Design review of the part built by this model. Coordinates are the model's own, in mm. Face numbers are marked on the shaded views. A direction names the side the tool comes from. Round coordinates to 2 decimals unless told otherwise and drop trailing zeros. Write each loop counter-clockwise with the first axis right and the second up, starting at its lowest first coordinate (ties: lowest second). Pieces come first, ordered by that corner, then holes.
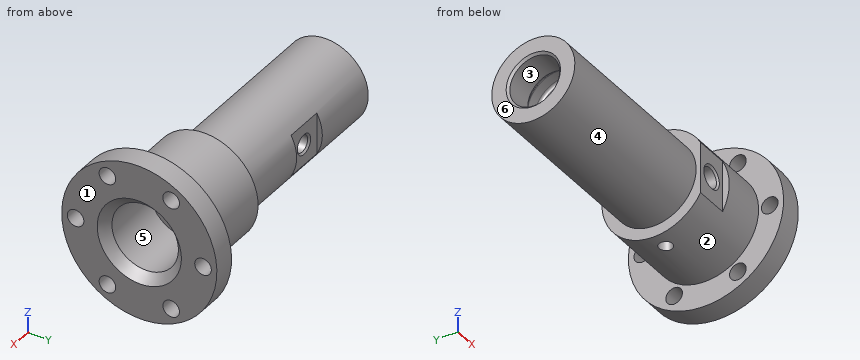
from build123d import *

# Parameters (mm, degrees)
FILLET2_R               = 2.5
SKETCH3_R               = 7.5
CUT_EXTRUDE1_DEPTH      = 274.541587332
CUT_EXTRUDE2_DEPTH      = 181.994025949
CUT_EXTRUDE2_DEPTH_BACK = 181.994025949
SKETCH4_W               = 35
SKETCH4_H               = 5
CUT_EXTRUDE3_DEPTH      = 181.994025949
CUT_EXTRUDE3_DEPTH_BACK = 181.994025949
SKETCH5_W               = 30
SKETCH5_H               = 6
SKETCH6_R               = 7.5
CUT_EXTRUDE4_DEPTH      = 28
SKETCH7_R               = 9
CUT_EXTRUDE5_DEPTH      = 33
CHAMFER6_SIZE           = 1.6
SKETCH8_R               = 6
CUT_EXTRUDE6_DEPTH      = 60


with BuildPart() as part:
    # Sketch1 → Revolve1 (revolve)
    with BuildSketch(Plane.XY, mode=Mode.PRIVATE) as revolve1_sk:
        Polygon((103.47826087, -30), (103.47826087, -70), (83.47826087, -70), (83.47826087, -47.5), (13.47826087, -47.5), (13.47826087, -37.5), (-151.52173913, -37.5), (-151.52173913, -22.5), (-125.02173913, -22.5), (-119.02173913, -27.5), (-106.52173913, -27.5), (-106.52173913, -17.5), (-16.52173913, -17.5), (-16.52173913, -27.5), (-1.52173913, -27.5), (-1.52173913, -22.5), (43.47826087, -22.5), (43.47826087, -30), align=None)
    revolve(revolve1_sk.sketch.rotate(Axis((-977.747346799, 0, 0), (1, 0, 0)), 270), axis=Axis((-977.747346799, 0, 0), (1, 0, 0)))

    # Fillet2
    fillet2_edges = [part.edges().sort_by_distance(p)[0] for p in [
        (-106.52173913, 0, -27.5),
        (-119.02173913, 0, -27.5),
    ]]
    fillet(fillet2_edges, radius=FILLET2_R)

    # Chamfer3: read off the stored shape, not the designer's step
    # Chamfer3 outline → Chamfer3 (revolve, cut)
    with BuildSketch(Plane.YX):
        Polygon((24.5, -151.52173913), (22.5, -149.52173913), (22.5, -151.52173913), align=None)
    revolve(axis=Axis((0, 0, 0), (1, 0, 0)), mode=Mode.SUBTRACT)

    # Chamfer4: read off the stored shape, not the designer's step
    # Chamfer4 outline → Chamfer4 (revolve, cut)
    with BuildSketch(Plane.YX):
        Polygon((30, 103.47826087), (30, 95.47826087), (38, 103.47826087), align=None)
    revolve(axis=Axis((0, 0, 0), (1, 0, 0)), mode=Mode.SUBTRACT)

    # Sketch3 → Cut-Extrude1 (cut, through all)
    with BuildSketch(Plane(origin=(103.47826087, 0, 0), x_dir=(0, 0, -1), z_dir=(1, 0, 0))):
        with Locations((0, 57.5)):
            Circle(SKETCH3_R)
        with Locations((49.796460718, 28.75)):
            Circle(SKETCH3_R)
        with Locations((49.796460718, -28.75)):
            Circle(SKETCH3_R)
        with Locations((0, -57.5)):
            Circle(SKETCH3_R)
        with Locations((-49.796460718, -28.75)):
            Circle(SKETCH3_R)
        with Locations((-49.796460718, 28.75)):
            Circle(SKETCH3_R)
    extrude(amount=-CUT_EXTRUDE1_DEPTH, mode=Mode.SUBTRACT)

    # Sketch4 → Cut-Extrude2 (cut, two sides: drawn at the far end of the back side and taken through both)
    with BuildSketch(Plane.XY.offset(-CUT_EXTRUDE2_DEPTH_BACK)):
        with Locations((-71.52173913, 35)):
            Rectangle(SKETCH4_W, SKETCH4_H)
    extrude(amount=CUT_EXTRUDE2_DEPTH + CUT_EXTRUDE2_DEPTH_BACK, mode=Mode.SUBTRACT)

    # Sketch5 → Cut-Extrude3 (cut, two sides: drawn at the far end of the back side and taken through both)
    with BuildSketch(Plane.XY.offset(-CUT_EXTRUDE3_DEPTH_BACK)):
        with Locations((28.47826087, -44.5)):
            Rectangle(SKETCH5_W, SKETCH5_H)
    extrude(amount=CUT_EXTRUDE3_DEPTH + CUT_EXTRUDE3_DEPTH_BACK, mode=Mode.SUBTRACT)

    # Sketch6 → Cut-Extrude4 (cut)
    with BuildSketch(Plane(origin=(0, 32.5, 0), x_dir=(1, 0, 0), z_dir=(0, 1, 0))):
        with Locations(Location((-71.52173913, 0, 0), (0, 0, 270))):
            Circle(SKETCH6_R)
    extrude(amount=-CUT_EXTRUDE4_DEPTH, mode=Mode.SUBTRACT)

    # Chamfer5: read off the stored shape, not the designer's step
    # Chamfer5 outline → Chamfer5 (revolve, cut)
    with BuildSketch(Plane(origin=(-71.52173913, 0, 0), x_dir=(1, 0, 0), z_dir=(0, 0, 1))):
        Polygon((7.5, 32.5), (7.5, 30.9), (9.1, 32.5), align=None)
    revolve(axis=Axis((-71.52173913, 0, 0), (0, 1, 0)), mode=Mode.SUBTRACT)

    # Sketch7 → Cut-Extrude5 (cut)
    with BuildSketch(Plane.XZ.offset(41.5)):
        with Locations(Location((28.47826087, 0, 0), (0, 0, 270))):
            Circle(SKETCH7_R)
    extrude(amount=-CUT_EXTRUDE5_DEPTH, mode=Mode.SUBTRACT)

    # Chamfer6
    chamfer6_edges = [part.edges().sort_by_distance(p)[0] for p in [
        (28.47826087, -41.5, 9),
    ]]
    chamfer(chamfer6_edges, length=CHAMFER6_SIZE)

    # Sketch8 → Cut-Extrude6 (cut)
    with BuildSketch(Plane.XY):
        with Locations((28.47826087, 0)):
            Circle(SKETCH8_R)
    extrude(amount=-CUT_EXTRUDE6_DEPTH, mode=Mode.SUBTRACT)


solid = part.part
1) For P1, Ø2, axis at x = 15, z = -34, coming from the -Y side; P2, Ø24, axis at x = 30, z = 1.5, coming from the -Y side; P3, Ø12, axis at x = -124.5, y = -15, coming from the +Z side; P4, Ø10, axis at x = -56.5, y = 45, coming from the -Z side, all flat-tipped, find the tip position at first contact; note any pin that passes through.
2) The part is to be moulded in two halves that separate along Y. For the marked faces 3, 4, 5 and 6, say which applies: pulls with the +Y half, pulls with the -Y half, needs draft (parallel to the pull), parting line crosses it, or undercut.
3) Add section A-A on x = -130.5. State the section outline as (y, z) points, and give its area (3 significant figures).
4) For the marked faces 1 and 2, list the 3-axis set-ups (+Z, -Z, +X, -X, +Y, -Y) from which the entire face can be reached by the end or side of a thin tool; tool diameter is ignored.
5) Add section C-C on y = 0. Count the separate pieces of the cut face and the enclosed holes in it, and give its area (3 significant figures).
6) Add section B-B on y = -57.5. State the section outline as (x, z) points, and give its area (3 significant figures).
7) For line 1 along Z through (x, y) = (-71, 25.5); line 2 along X through (y, z) = (25, -1.5); line 3 along X through (y, z) = (23, 0), list the stretches that pass through material, from the lowest coordinate up.
Computed:
1. P1: stops at y = -34.17
1. P2: stops at y = -41.5
1. P3: stops at z = 36.4
1. P4: passes through
2. face 3: undercut
2. face 4: parting line crosses it
2. face 5: undercut
2. face 6: needs draft
3. outline: circle Ø75 at (0, 0); hole circle Ø45 at (0, 0)
3. area: 2,830 mm2
4. face 1: +Z, -Z, +X, +Y, -Y
4. face 2: -X
5. separate pieces: 3
5. enclosed holes: 0
5. area: 9,680 mm2
6. outline: (83.48, -39.92) - (103.48, -39.92) - (103.48, -7.5) - (83.48, -7.5) - close; (83.48, 7.5) - (103.48, 7.5) - (103.48, 39.92) - (83.48, 39.92) - close
6. area: 1,300 mm2
7. line 1: z = -27.5 to -7.48, 7.48 to 27.5
7. line 2: x = -151.52 to -121.97, -106.52 to -78.87, -64.17 to -16.52, -1.52 to 43.48
7. line 3: x = -150.02 to -124.42, -106.52 to -79.02, -64.02 to -16.52, -1.52 to 43.48
